For this review, take the finished solid that the model builds, in its own axes (mm). A direction names the side the tool comes from. Round coordinates to 2 decimals unless told otherwise and drop trailing zeros. Loops run counter-clockwise (first coordinate to the right, second up) from the corner with the lowest first, then second, coordinate; pieces in that order, holes last.
1) Insertion check: pin 1 (0.8 mm diameter, centred on x = -11.5, z = -11.5, fed in from -Y); pin 2 (3.5 mm diameter, centred on x = 0, y = 5, fed in from +Z). Each pin has a flat end and moves straight along its axis. Give the tip position at first contact, or say it passes through.
2) Wall thickness on L1, parallel to X at y = 4, z = 0; L2, parallel to Z at x = 1, y = 9; L3, parallel to X at y = 2.75, z = -2: over which ranges is each line inside the solid? List them lowest first.
3) Mouldability with a two-part tool opening along X and no side actions: class faces 3 (the cylindrical face through (0, 5, -5)), 4 (the flat face through (-0.3, 10, -5.3)), 5 (the cylindrical face through (-24.715, 5.056, 14.699)), 6 (the cylindrical face through (10.582, 2.465, 11.476)) as pulls with the +X half, pulls with the -X half, needs draft (parallel to the pull), parting line crosses it, or undercut.
4) Take a section at B-B (z = 0). State the section outline as (x, y) points.
5) Tool access review of faces 1 (the cylindrical face through (0.336, 9.699, -24.715)), 2 (the cylindrical face through (-10.81, 2.46, -10.76)): name each direction out of +Z, -Z, +X, -X, +Y, -Y from which nothing blocks a thin tool from reaching the whole face with its end or side.
6) Take a section at A-A (x = 0). State the section outline as (y, z) points, then the cut area to 3 significant figures.
7) Take a section at C-C (z = 8). State the section outline as (x, y) points, then the cut area to 3 significant figures.
```python
from build123d import *

# Parameters (mm, degrees)
SKETCH1_W               = 50
SKETCH1_H               = 40
SKETCH1_R               = 5
BOSS_EXTRUDE1_DEPTH     = 10
SKETCH2_R               = 0.75
CUT_EXTRUDE1_DEPTH      = 5
CUT_EXTRUDE2_REACH      = 50.218
CUT_EXTRUDE2_END_RADIUS = 5
SKETCH3_R               = 2
FILLET1_R               = 1


with BuildPart() as part:
    # Sketch1 → Boss-Extrude1 (new body)
    with BuildSketch(Plane(origin=(0, 0, 0), x_dir=(1, 0, 0), z_dir=(0, 1, 0))):
        with Locations((0, 5)):
            Rectangle(SKETCH1_W, SKETCH1_H)
        with Locations(Location((0, 0, 0), (0, 0, 270))):
            Circle(SKETCH1_R, mode=Mode.SUBTRACT)
    extrude(amount=BOSS_EXTRUDE1_DEPTH)

    # Sketch2 → Cut-Extrude1 (cut)
    with BuildSketch(Plane.XZ):
        with Locations(Location((-11.313708499, 11.313708499, 0), (0, 0, 270))):
            Circle(SKETCH2_R)
        with Locations(Location((11.313708499, 11.313708499, 0), (0, 0, 270))):
            Circle(SKETCH2_R)
        with Locations(Location((11.313708499, -11.313708499, 0), (0, 0, 270))):
            Circle(SKETCH2_R)
        with Locations(Location((-11.313708499, -11.313708499, 0), (0, 0, 270))):
            Circle(SKETCH2_R)
    extrude(amount=-CUT_EXTRUDE1_DEPTH, mode=Mode.SUBTRACT)

    # Cut-Extrude2: up to this cylinder (the profile starts outside it)
    cut_extrude2_end = Plane(origin=(0, 5, 0), z_dir=(0, -1, 0)) * Cylinder(CUT_EXTRUDE2_END_RADIUS, 111.436, mode=Mode.PRIVATE)
    # Sketch3 → Cut-Extrude2 (cut, up to the surface)
    with BuildSketch(Plane.XY.offset(15), mode=Mode.PRIVATE) as cut_extrude2_sk1:
        with Locations((0, 5)):
            Circle(SKETCH3_R)
    cut_extrude2_tool1 = extrude(cut_extrude2_sk1.sketch, amount=-CUT_EXTRUDE2_REACH, mode=Mode.PRIVATE) - cut_extrude2_end
    add(cut_extrude2_tool1.solids().sort_by_distance((0, 5, 15))[0], mode=Mode.SUBTRACT)

    # Fillet1
    fillet1_edges = [part.edges().sort_by_distance(p)[0] for p in [
        (-25, 10, -5),
        (0, 10, 15),
        (25, 10, -5),
        (0, 0, 15),
        (-25, 0, -5),
        (0, 0, -25),
        (25, 0, -5),
        (25, 5, 15),
        (-25, 5, 15),
        (-25, 5, -25),
        (25, 5, -25),
        (0, 10, -25),
    ]]
    fillet(fillet1_edges, radius=FILLET1_R)


solid = part.part
```
Response:
1. pin 1: stops at y = 5
1. pin 2: stops at z = -4.68
2. L1: x = -25 to -5, 5 to 25
2. L2: z = -25 to -4.9, 4.9 to 15
2. L3: x = -25 to -4.58, 4.58 to 25
3. face 3: undercut
3. face 4: needs draft
3. face 5: pulls with the -X half
3. face 6: undercut
4. outline: (-25, 1) arc R1 ccw to (-24, 0) - (-5, 0) - (-5, 10) - (-24, 10) arc R1 ccw to (-25, 9) - close; (5, 0) - (24, 0) arc R1 ccw to (25, 1) - (25, 9) arc R1 ccw to (24, 10) - (5, 10) - close
5. face 1: -Z, +X, -X, +Y
5. face 2: -Y
6. outline: (0, -24) arc R1 ccw to (1, -25) - (9, -25) arc R1 ccw to (10, -24) - (10, -5) - (0, -5) - close; (0, 5) - (3, 5) - (3, 15) - (1, 15) arc R1 ccw to (0, 14) - close; (7, 5) - (10, 5) - (10, 14) arc R1 ccw to (9, 15) - (7, 15) - close
6. area: 259 mm2
7. outline: (-25, 1) arc R1 ccw to (-24, 0) - (24, 0) arc R1 ccw to (25, 1) - (25, 9) arc R1 ccw to (24, 10) - (-24, 10) arc R1 ccw to (-25, 9) - close; hole circle Ø4 at (0, 5)
7. area: 487 mm2
